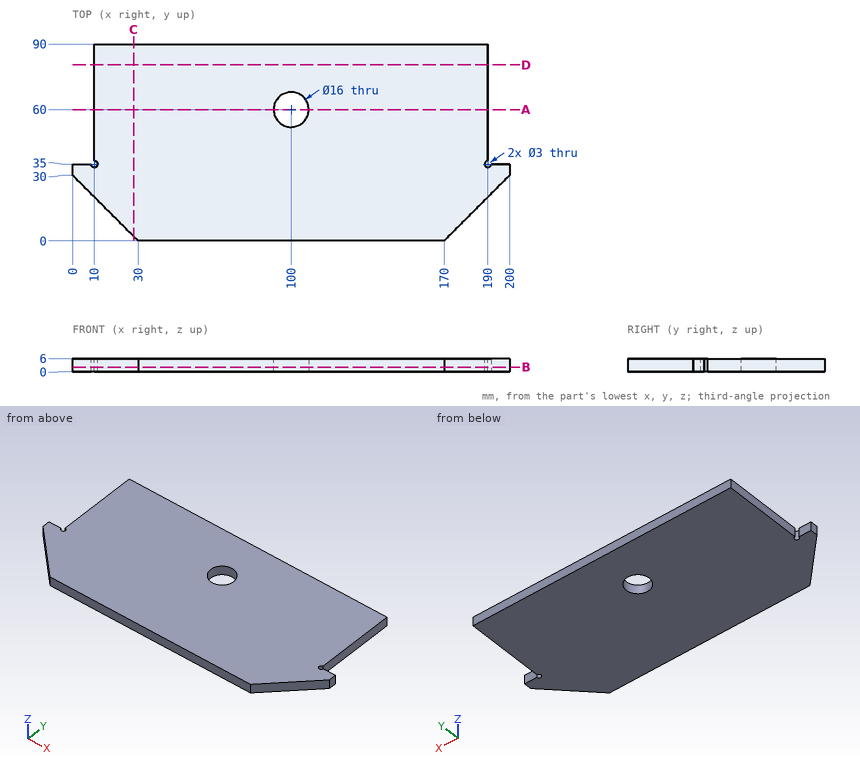
Answer from the drawing. Dimensions are ordinates in mm from the lowest x, y and z of the part. Coordinates: 2 decimals unless noted, no trailing zeros. Write each loop counter-clockwise with the first axis right and the second up, starting at its lowest first coordinate (ties: lowest second). Pieces come first, ordered by that corner, then holes. Notation, with made-up numbers: M 45.5,-18 L 54.5,-18 A19 ccw 54.5,-9 Z; hole C 17.5,64 d4. An arc over 180 degrees is marked long. Use one line per item in the form item = value. Start each with the question number.
1. The part is cut by section C-C (x = 28). Give the vertices of the cut face in (y, z).
2. The part is cut by section D-D (y = 80.5). Give the vertices of the cut face in (x, z), plus the area to 3 significant figures.
3. Straight lines are drawn through the part: probe 1 along Y at (x, z) = (100, 3.55); probe 2 along X at (y, z) = (60, 2.8); probe 3 along X at (y, z) = (34.5, 1.9). For each, find the intervals that lie inside material, in ascending order. Write a range as from..to.
4. The part is cut by section A-A (y = 60). Give the vertices of the cut face in (x, z), plus the area to 3 significant figures.
5. The part is cut by section B-B (z = 2.2). Give the vertices of the cut face in (x, y), plus the area to 3 significant figures.
6. Each of these flat-tipped pins is pushed along its axis until it touches: P1, Ø4, axis at x = 190, y = 35, coming from the +Z side; P2, Ø1, axis at x = 179.5, z = 3, coming from the -Y side; P3, Ø1.8, axis at y = 54.5, z = 4, coming from the +X side. Where does it stop, or does it pass through?
Evaluation:
q1.outline = M 2,0 L 90,0 L 90,6 L 2,6 Z
q2.outline = M 10,0 L 190,0 L 190,6 L 10,6 Z
q2.area = 1,080 mm^2
q3.probe_1 = 0..52, 68..90
q3.probe_2 = 10..92, 108..190
q3.probe_3 = 0..8.59, 11.41..188.59, 191.41..200
q4.outline = M 10,0 L 92,0 L 92,6 L 10,6 Z; M 108,0 L 190,0 L 190,6 L 108,6 Z
q4.area = 984 mm^2
q5.outline = M 0,30 L 30,0 L 170,0 L 200,30 L 200,35 L 191.5,35 A1.5 cw long 190,36.5 L 190,90 L 10,90 L 10,36.5 A1.5 cw long 8.5,35 L 0,35 Z; hole C 100,60 d16
q5.area = 15,800 mm^2
q6.P1 = 6
q6.P2 = 9
q6.P3 = 190
